Design review of the part built by this model. Coordinates are the model's own, in mm. A direction names the side the tool comes from. Round coordinates to 2 decimals unless told otherwise and drop trailing zeros. Loops run counter-clockwise (first coordinate to the right, second up) from the corner with the lowest first, then second, coordinate; pieces in that order, holes last. Notation, with made-up numbers: (-23.5, 43.5) - (21.5, 43.5) arc R29 ccw to (21.5, 73.5) - close; hole circle Ø4 at (43, 31). An arc over 180 degrees is marked (long way). Use one line per item in the form item = value. Start each with the question number.
(1) Wall thickness on probe 1 along Z at (x, y) = (10, 111); probe 2 along X at (y, z) = (274.32, -12): over which ranges is each line inside the solid? List them lowest first. Write a range as [from, to].
(2) Machinability: for faces 1 (the cylindrical face through (0.553, 271.828, -11.917)), 2 (the flat face through (0, 142, -11.112)), which of the approach directions +Z, -Z, +X, -X, +Y, -Y give a long, thin tool a straight path to every point of the face, cutting with its end or side? Answer none if there is none.
(3) We need section C-C, the plane x = -7.5. Write out the cut boundary in (y, z).
(4) We need section B-B, the plane y = 217.5. Write out the cut boundary in (x, z), then the cut area to 3 significant figures.
(5) For pin 1 (4.5 mm diameter, centred on x = 0, y = 63.5, fed in from -Z), flat-tipped, find the tip position at first contact; note if it passes through.
(6) We need section D-D, the plane y = 105.41. Write out the cut boundary in (x, z).
(7) We need section A-A, the plane z = 2. Write out the cut boundary in (x, y).
(8) The part is to be moulded in two halves that separate along Z. For faces 3 (the flat face through (0, 142, -12.7)), 4 (the flat face through (0, 142, 12.7)), 5 (the cylindrical face through (0.553, 10.208, 11.895)), 6 (the flat face through (-11.112, 142, 0)), say which applies: released by +Z, released by -Z, zero draft, split by the parting line, or undercut.
from build123d import *

# Parameters (mm, degrees)
SKETCH1_W                        = 25.4
SKETCH1_H                        = 25.4
SKETCH1_W_2                      = 22.225
SKETCH1_H_2                      = 22.225
BOSS_EXTRUDE1_DEPTH              = 287.02
F_10_CLEARANCE_HOLE1_D           = 5.1054
F_13_64_0_20313_DIAMETER_HOLE1_D = 5.159502


with BuildPart() as part:
    # Sketch1 → Boss-Extrude1 (new body)
    with BuildSketch(Plane(origin=(0, 0, 0), x_dir=(1, 0, 0), z_dir=(0, 1, 0))):
        Rectangle(SKETCH1_W, SKETCH1_H)
        Rectangle(SKETCH1_W_2, SKETCH1_H_2, mode=Mode.SUBTRACT)
    extrude(amount=BOSS_EXTRUDE1_DEPTH)

    # #10 Clearance Hole1 (through all)
    with Locations(Plane.XY.offset(12.7)):
        with Locations((0, 274.32), (0, 248.92), (0, 223.52), (0, 63.5), (0, 38.1), (0, 12.7)):
            Hole(F_10_CLEARANCE_HOLE1_D / 2)

    # 13/64 (0.20313) Diameter Hole1 (through all)
    with Locations(Plane(origin=(-522.170199168, -199.39, -12.7), x_dir=(0, 1, 0), z_dir=(0, 0, -1))):
        with Locations((304.8, 522.170199168), (381, 522.170199168)):
            Hole(F_13_64_0_20313_DIAMETER_HOLE1_D / 2)


solid = part.part
Data:
q1.probe_1 = [-12.7, -11.11], [11.11, 12.7]
q1.probe_2 = [-12.7, -2.55], [2.55, 12.7]
q2.face_1 = +Z, -Z
q2.face_2 = +Y, -Y
q3.outline = (0, -12.7) - (287.02, -12.7) - (287.02, -11.11) - (0, -11.11) - close; (0, 11.11) - (287.02, 11.11) - (287.02, 12.7) - (0, 12.7) - close
q4.outline = (-12.7, -12.7) - (12.7, -12.7) - (12.7, 12.7) - (-12.7, 12.7) - close; hole (-11.11, -11.11) - (11.11, -11.11) - (11.11, 11.11) - (-11.11, 11.11) - close
q4.area = 151 mm^2
q5.pin_1 = through
q6.outline = (-12.7, -12.7) - (-2.58, -12.7) - (-2.58, -11.11) - (-11.11, -11.11) - (-11.11, 11.11) - (-2.58, 11.11) - (-2.58, 12.7) - (-12.7, 12.7) - close; (2.58, -12.7) - (12.7, -12.7) - (12.7, 12.7) - (2.58, 12.7) - (2.58, 11.11) - (11.11, 11.11) - (11.11, -11.11) - (2.58, -11.11) - close
q7.outline = (-12.7, 0) - (-11.11, 0) - (-11.11, 287.02) - (-12.7, 287.02) - close; (11.11, 0) - (12.7, 0) - (12.7, 287.02) - (11.11, 287.02) - close
q8.face_3 = released by -Z
q8.face_4 = released by +Z
q8.face_5 = zero draft
q8.face_6 = undercut
